Geometry check sheet. Reference: the model listing, model coordinates, mm. Face numbers are marked on the shaded views. A direction names the side the tool comes from. Coordinates: 2 decimals unless noted, no trailing zeros. Write each loop counter-clockwise with the first axis right and the second up, starting at its lowest first coordinate (ties: lowest second). Pieces come first, ordered by that corner, then holes. Notation, with made-up numbers: (54, -26.5) -> (108, -26.5) arc R29 ccw to (108, -0.5) -> close; hole circle Ø9 at (-5.5, 48). An arc over 180 degrees is marked (long way). Use a Markdown table: item, result.
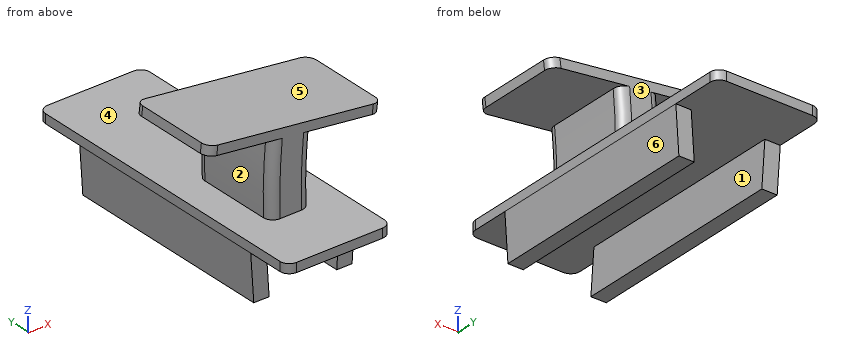
```python
from build123d import *

# Parameters (mm, degrees)
F0_W     = 34
F0_H     = 102
F1_DEPTH = 3
F6_W     = 57
F6_H     = 30
F7_DEPTH = 3
F8_R     = 3
F2_W     = 5
F2_H     = 70
F10_W    = 5
F10_H    = 70
F13_R    = 3


# Not quite as in the source:
# - a feature names something its author has since deleted; it is built from what else it names


with BuildPart() as f1:
    # F0 (on Top) → F1 (new body)
    with BuildSketch(Plane.XY):
        with Locations((0, 1)):
            Rectangle(F0_W, F0_H)
    extrude(amount=F1_DEPTH)

    # F5: sweep along a path in F4
    with BuildLine(Plane.XZ) as f5_path:
        ThreePointArc((0.7317709574, 26), (0.0173632461, 14.5110886282), (0, 3))
    # F3 (on face) → F5 (sweep)
    with BuildSketch(Plane.XY.offset(3)):
        Polygon((6.5, 0), (0, 0), (-6.5, 0), (-6.5, -30), (0, -30), (6.5, -30), align=None)
    sweep(path=f5_path.line)

    # F6 (on face) → F7 (join)
    with BuildSketch(Plane(origin=(3.1308235326, 0, 25.7078318269), x_dir=(0.9926657135, 0, -0.1208916099), z_dir=(0.1208916099, 0, 0.9926657135))):
        with Locations((-1.916777917, -15)):
            Rectangle(F6_W, F6_H)
    extrude(amount=F7_DEPTH)

    # F8
    f8_edges = [f1.edges().sort_by_distance(p)[0] for p in [
        (29.700414, -30, 23.983142),
        (29.700414, 0, 23.983142),
        (-26.881532, -30, 30.873964),
        (-26.881532, 0, 30.873964),
    ]]
    fillet(f8_edges, radius=F8_R)

    # F2 (on face) → F11 section 0
    with BuildSketch(Plane(origin=(0, 0, 0), x_dir=(1, 0, 0), z_dir=(0, 0, -1))):
        with Locations((14.5, 0)):
            Rectangle(F2_W, F2_H)
    # F10 (on offset) → F11 section 1
    with BuildSketch(Plane.XY.offset(-15)):
        with Locations((13.5, 0)):
            Rectangle(F10_W, F10_H)
    loft()

    # F2 (on face) → F12 section 0
    with BuildSketch(Plane(origin=(0, 0, 0), x_dir=(1, 0, 0), z_dir=(0, 0, -1))):
        with Locations((-14.5, 0)):
            Rectangle(F2_W, F2_H)
    # F10 (on offset) → F12 section 1
    with BuildSketch(Plane.XY.offset(-15)):
        with Locations((-13.5, 0)):
            Rectangle(F10_W, F10_H)
    loft()

    # F13
    f13_edges = [f1.edges().sort_by_distance(p)[0] for p in [
        (17, -50, 1.5),
        (-17, -50, 1.5),
        (17, 52, 1.5),
        (-17, 52, 1.5),
        (6.505434, -30, 14.117469),
        (-6.470708, -30, 14.904709),
        (6.505434, 0, 14.117469),
        (-6.470708, 0, 14.904709),
    ]]
    fillet(f13_edges, radius=F13_R)


solid = f1.part
```
Item 1: Section check A-A on y = -25. Record the boundary of the cut face in (x, z).
Answer block:
| item | result |
|---|---|
| outline | (-27.06, 29.38) -> (-5.72, 26.79) arc R196.5 ccw to (-6.5, 3) -> (-17, 3) -> (-17, 0) -> (-16, -15) -> (-11, -15) -> (-12, 0) -> (12, 0) -> (11, -15) -> (16, -15) -> (17, 0) -> (17, 3) -> (6.5, 3) arc R183.5 cw to (7.18, 25.21) -> (29.52, 22.49) -> (29.88, 25.47) -> (-26.7, 32.36) -> close |
Item 2: Tool access check on the marked faces 1, 2 and 3. Record the directions out of +Z, -Z, +X, -X, +Y, -Y that give a thin tool (end or side, any length) a straight path to the whole face; none if there is none.
Answer block:
| item | result |
|---|---|
| face 1 | +Y, -Y |
| face 2 | -X, +Y, -Y |
| face 3 | +Z, +X, -X, +Y |
Item 3: Thickness scan on L1, parallel to X at y = 18, z = -2; L2, parallel to Y at x = 1, z = 23; L3, parallel to X at y = 15, z = 0.5. Record the ranges inside material, lowest first. Write a range as [from, to].
Answer block:
| item | result |
|---|---|
| L1 | x = [-16.87, -11.87], [11.87, 16.87] |
| L2 | y = [-30, 0] |
| L3 | x = [-17, 17] |
Item 4: Section check B-B on x = 2. Record the boundary of the cut face in (y, z), then the cut area to 3 significant figures.
Answer block:
| item | result |
|---|---|
| outline | (-50, 0) -> (52, 0) -> (52, 3) -> (0, 3) -> (0, 28.87) -> (-30, 28.87) -> (-30, 3) -> (-50, 3) -> close |
| area | 1,080 mm^2 |
Item 5: Section check C-C on y = 22. Record the boundary of the cut face in (x, z).
Answer block:
| item | result |
|---|---|
| outline | (-17, 0) -> (-16, -15) -> (-11, -15) -> (-12, 0) -> (12, 0) -> (11, -15) -> (16, -15) -> (17, 0) -> (17, 3) -> (-17, 3) -> close |
Item 6: Section check D-D on x = 23. Record the boundary of the cut face in (y, z), then the cut area to 3 significant figures.
Answer block:
| item | result |
|---|---|
| outline | (-30, 23.29) -> (0, 23.29) -> (0, 26.31) -> (-30, 26.31) -> close |
| area | 90.7 mm^2 |
Item 7: Depth check by flat-ended pin: P1, Ø3.5, axis at y = 3.5, z = 1, coming from the -X side; P2, Ø2.5, axis at y = -7.5, z = 1.5, coming from the +X side; P3, Ø8, axis at x = 14.5, y = -29.5, coming from the +Z side; P4, Ø10, axis at x = 2.5, z = -7, coming from the -Y side. Enter the tip coordinate at first touch or a pass-through.
Answer block:
| item | result |
|---|---|
| P1 | stops at x = -17 |
| P2 | stops at x = 17 |
| P3 | stops at z = 27.83 |
| P4 | passes through |
Item 8: Mould release check, pull along Z, two halves, no side actions. Record for the marked faces 4, 5 and 6: +Z half, -Z half, draft (parallel to the pull), parting line (faces both ways), or undercut.
Answer block:
| item | result |
|---|---|
| face 4 | undercut |
| face 5 | +Z half |
| face 6 | -Z half |
